```python
from build123d import *

# Parameters (mm, degrees)
SKETCH1_R                    = 241.3
SKETCH1_R_2                  = 190.5
SKETCH1_R_3                  = 12.7
BOSS_EXTRUDE1_DEPTH          = 25.4
SKETCH19_W                   = 762
SKETCH19_H                   = 609.6
BASE_FLANGE1_DEPTH           = 6
EDGE_FLANGE1_STRIP_CUT_DEPTH = 609.6
EDGE_FLANGE1_DEPTH           = 609.6
EDGE_FLANGE2_STRIP_W         = 25.4732
EDGE_FLANGE2_STRIP_H         = 6
EDGE_FLANGE2_STRIP_CUT_DEPTH = 609.6
EDGE_FLANGE2_DEPTH           = 609.6
BOSS_EXTRUDE2_DEPTH          = 12.7
BOSS_EXTRUDE2_DEPTH_BACK     = 12.7
FILLET1_R                    = 76.2
SKETCH30_R                   = 12.7
CUT_EXTRUDE1_DEPTH           = 783.174585068
FILLET3_R                    = 76.2


# Sheet-metal steps are written as plain solids
with BuildPart() as part:
    # Sketch1 → Boss-Extrude1 (new body)
    with BuildSketch(Plane.XY):
        Circle(SKETCH1_R)
        Circle(SKETCH1_R_2, mode=Mode.SUBTRACT)
        with Locations((55.879031838, 208.543385896)):
            Circle(SKETCH1_R_3, mode=Mode.SUBTRACT)
        with Locations((152.664354058, 152.664354058)):
            Circle(SKETCH1_R_3, mode=Mode.SUBTRACT)
        with Locations((208.543385896, 55.879031838)):
            Circle(SKETCH1_R_3, mode=Mode.SUBTRACT)
        with Locations((208.543385896, -55.879031838)):
            Circle(SKETCH1_R_3, mode=Mode.SUBTRACT)
        with Locations((152.664354058, -152.664354058)):
            Circle(SKETCH1_R_3, mode=Mode.SUBTRACT)
        with Locations((55.879031838, -208.543385896)):
            Circle(SKETCH1_R_3, mode=Mode.SUBTRACT)
        with Locations((-55.879031838, -208.543385896)):
            Circle(SKETCH1_R_3, mode=Mode.SUBTRACT)
        with Locations((-152.664354058, -152.664354058)):
            Circle(SKETCH1_R_3, mode=Mode.SUBTRACT)
        with Locations((-208.543385896, -55.879031838)):
            Circle(SKETCH1_R_3, mode=Mode.SUBTRACT)
        with Locations((-208.543385896, 55.879031838)):
            Circle(SKETCH1_R_3, mode=Mode.SUBTRACT)
        with Locations((-152.664354058, 152.664354058)):
            Circle(SKETCH1_R_3, mode=Mode.SUBTRACT)
        with Locations((-55.879031838, 208.543385896)):
            Circle(SKETCH1_R_3, mode=Mode.SUBTRACT)
    extrude(amount=BOSS_EXTRUDE1_DEPTH)



with BuildPart() as body_2:
    # Sketch19 → Base-Flange1 (new body)
    with BuildSketch(Plane(origin=(0, -317.5, 0), x_dir=(1, 0, 0), z_dir=(0, 1, 0))):
        with Locations((0, -12.7)):
            Rectangle(SKETCH19_W, SKETCH19_H)
    extrude(amount=-BASE_FLANGE1_DEPTH)

    # Edge-Flange1 strip (across the edge) → Edge-Flange1 strip cut (cut)
    with BuildSketch(Plane(origin=(381, -317.5, 317.5), x_dir=(-0.7071067811865438, 0.7071067811865512, 0), z_dir=(0, 0, -1))):
        Polygon((-22.039168001, 13.553886626), (-4.026895542, -4.458385832), (0.215745145, -0.215745145), (-17.796527314, 17.796527314), align=None)
    extrude(amount=EDGE_FLANGE1_STRIP_CUT_DEPTH, mode=Mode.SUBTRACT)

    # Edge-Flange1 section (across the edge) → Edge-Flange1 (add)
    with BuildSketch(Plane(origin=(381, -317.5, 317.5), x_dir=(-0.7071067811865438, 0.7071067811865512, 0), z_dir=(0, 0, -1))):
        with BuildLine():
            Line((-6, 0.30510971), (-6, 356.670718626))
            Line((-6, 356.670718626), (0, 356.670718626))
            Line((0, 356.670718626), (0, 0.30510971))
            ThreePointArc((0, 0.30510971), (0.056070336, 0.023225094), (0.215745145, -0.215745145))
            Line((0.215745145, -0.215745145), (-4.026895542, -4.458385832))
            ThreePointArc((-4.026895542, -4.458385832), (-5.487206859, -2.2728755), (-6, 0.30510971))
        make_face()
    extrude(amount=EDGE_FLANGE1_DEPTH)

    # Edge-Flange2 strip (across the edge) → Edge-Flange2 strip cut (cut)
    with BuildSketch(Plane(origin=(-381, -317.5, -292.1), x_dir=(1, 0, 0), z_dir=(0, 0, 1))):
        with Locations((-12, -3)):
            Rectangle(EDGE_FLANGE2_STRIP_W, EDGE_FLANGE2_STRIP_H)
    extrude(amount=EDGE_FLANGE2_STRIP_CUT_DEPTH, mode=Mode.SUBTRACT)

    # Edge-Flange2 section (across the edge) → Edge-Flange2 (add)
    with BuildSketch(Plane(origin=(-381, -317.5, -292.1), x_dir=(1, 0, 0), z_dir=(0, 0, 1))):
        with BuildLine():
            Line((-6, 0.7366), (-6, 248))
            Line((-6, 248), (0, 248))
            Line((0, 248), (0, 0.7366))
            ThreePointArc((0, 0.7366), (0.215745145, 0.215745145), (0.7366, 0))
            Line((0.7366, 0), (0.7366, -6))
            ThreePointArc((0.7366, -6), (-4.026895542, -4.026895542), (-6, 0.7366))
        make_face()
    extrude(amount=EDGE_FLANGE2_DEPTH)


with BuildPart() as part_1:
    add(part.part)

    add(body_2.part)  # Boss-Extrude2 merges body 2
    # Sketch2 → Boss-Extrude2 (add, two sides: drawn at the far end of the back side and taken through both)
    with BuildSketch(Plane(origin=(0, 0, 12.7), x_dir=(-1, 0, 0), z_dir=(0, 0, -1)).offset(-BOSS_EXTRUDE2_DEPTH_BACK)):
        with BuildLine():
            Line((-176.371629871, 164.677679655), (-508, -190.5))
            Line((-508, -190.5), (-381, -317.5))
            Line((-381, -317.5), (381, -317.5))
            Line((381, -317.5), (381, -190.5))
            Line((381, -190.5), (211.187529283, 116.728391899))
            ThreePointArc((211.187529283, 116.728391899), (-29.628031694, -239.474152547), (-176.371629871, 164.677679655))
        make_face()
    extrude(amount=BOSS_EXTRUDE2_DEPTH + BOSS_EXTRUDE2_DEPTH_BACK)

    # Fillet1
    # the kernel refuses this fillet: 76.2 mm, written as the material it adds along each edge
    with BuildSketch(Plane(origin=(-381, -190.5, 0), x_dir=(0, 1, 0), z_dir=(0, 0, 1))) as fillet1_piece_1:
        with BuildLine():
            CenterArc((194.419807723, -20.395387566), FILLET1_R, 164.475167034, 76.594355804)
            Line((157.558210281, -87.086186287), (156.820978332, -88.420002261))
            Line((156.820978332, -88.420002261), (-0.737231949, -1.333815974))
            Line((-0.737231949, -1.333815974), (0, 1.524))
            ThreePointArc((0, 1.524), (60.5, 1.524), (119.531603846, 0.407907751))
            Line((119.531603846, 0.407907751), (121, 0))
        make_face()
    extrude(amount=25.4)
    with BuildSketch(Plane(origin=(508, -190.5, 25.4), x_dir=(0.7071067811865509, 0.707106781186544, 0), z_dir=(0, 0, -1))) as fillet1_piece_2:
        with BuildLine():
            CenterArc((FILLET1_R * 1.03487581695, -FILLET1_R), FILLET1_R, 90, 91.963796982)
            Line((FILLET1_R * 0.0354631377737, -FILLET1_R * 1.03426801283), (FILLET1_R * 0.0154748841901, -FILLET1_R * 1.03495337309))
            Line((FILLET1_R * 0.0154748841901, -FILLET1_R * 1.03495337309), (-FILLET1_R * 0.020697516339, FILLET1_R * 0.02))
            Line((-FILLET1_R * 0.020697516339, FILLET1_R * 0.02), (FILLET1_R * 1.03487581695, FILLET1_R * 0.02))
            Line((FILLET1_R * 1.03487581695, FILLET1_R * 0.02), (FILLET1_R * 1.03487581695, 0))
        make_face()
    extrude(amount=25.4)

    # Sketch30 → Cut-Extrude1 (cut, through all)
    # profile 1 of 3: a face of its own
    with BuildSketch(Plane(origin=(0, 0, 0), x_dir=(-1, 0, 0), z_dir=(0, 0, -1))):
        with BuildLine():
            Line((-330.130702101, 0), (-241.3, 0))
            ThreePointArc((-241.3, 0), (-224.481808047, 88.507671171), (-176.371629871, 164.677679655))
            Line((-176.371629871, 164.677679655), (-330.130702101, 0))
        make_face()
    # profile 2 of 3: a face of its own
    with BuildSketch(Plane(origin=(0, 0, 0), x_dir=(-1, 0, 0), z_dir=(0, 0, -1))):
        with BuildLine():
            Line((-241.3, 0), (-190.5, 0))
            ThreePointArc((-190.5, 0), (0, 190.5), (190.5, 0))
            Line((190.5, 0), (241.3, 0))
            ThreePointArc((241.3, 0), (233.650637508, 60.274949954), (211.187529283, 116.728391899))
            ThreePointArc((211.187529283, 116.728391899), (29.628031694, 239.474152547), (-176.371629871, 164.677679655))
            ThreePointArc((-176.371629871, 164.677679655), (-224.481808047, 88.507671171), (-241.3, 0))
        make_face()
        with Locations((-208.543385896, 55.879031838)):
            Circle(SKETCH30_R, mode=Mode.SUBTRACT)
        with Locations((-152.664354058, 152.664354058)):
            Circle(SKETCH30_R, mode=Mode.SUBTRACT)
        with Locations((-55.879031838, 208.543385896)):
            Circle(SKETCH30_R, mode=Mode.SUBTRACT)
        with Locations((208.543385896, 55.879031838)):
            Circle(SKETCH30_R, mode=Mode.SUBTRACT)
        with Locations((55.879031838, 208.543385896)):
            Circle(SKETCH30_R, mode=Mode.SUBTRACT)
        with Locations((152.664354058, 152.664354058)):
            Circle(SKETCH30_R, mode=Mode.SUBTRACT)
    # profile 3 of 3: a face of its own
    with BuildSketch(Plane(origin=(0, 0, 0), x_dir=(-1, 0, 0), z_dir=(0, 0, -1))):
        with BuildLine():
            ThreePointArc((211.187529283, 116.728391899), (233.650637508, 60.274949954), (241.3, 0))
            Line((241.3, 0), (275.706099682, 0))
            Line((275.706099682, 0), (211.187529283, 116.728391899))
        make_face()
    extrude(amount=-CUT_EXTRUDE1_DEPTH, mode=Mode.SUBTRACT)

    # Fillet3
    fillet3_edges = [part_1.edges().sort_by_distance(p)[0] for p in [
        (-275.706099682, 0, 12.7),
        (330.130702101, 0, 12.7),
    ]]
    fillet(fillet3_edges, radius=FILLET3_R)


solid = part_1.part
```
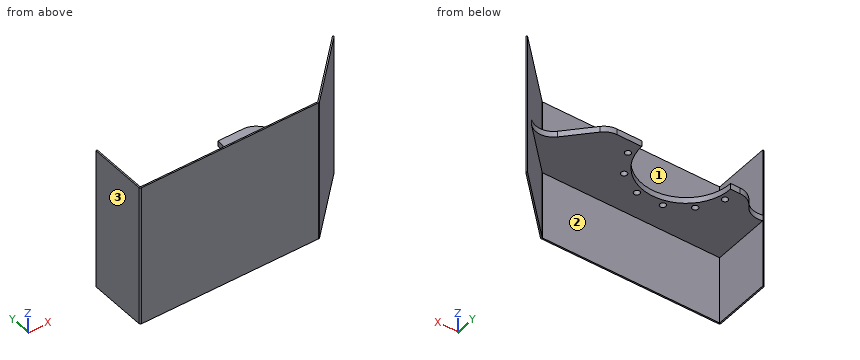
CAD build for the part. Positions are in the model's coordinates, mm. Face numbers are marked on the shaded views. A direction names the side the tool comes from. Coordinates: 2 decimals unless noted, no trailing zeros. Order: outer loops, then holes, each group sorted by start corner. A loop starts at its lowest first (then second) coordinate and runs counter-clockwise, first axis right, second up.
(1) Which spindle directions (+Z, -Z, +X, -X, +Y, -Y) get a long thin tool onto all of the face, cutting with end or side? Do the marked faces 1, 2 and 3. Say none if no direction does.
Solution:
face 1: +Z, +Y
face 2: -Z, +Y
face 3: +Z, -Z, -X, +Y, -Y
(2) Saw through at A-A, the plane x = 0. Write the cut outline in (y, z).
Solution:
outline: (-323.5, -292.1) - (-317.5, -292.1) - (-317.5, 0) - (-190.5, 0) - (-190.5, 25.4) - (-317.5, 25.4) - (-317.5, 317.5) - (-323.5, 317.5) - close
(3) Saw through at C-C, the plane x = 477.5. Write the cut outline in (y, z), and give its area (3 significant figures).
Solution:
outline: (-229.49, -292.1) - (-221, -292.1) - (-221, 0) - (-149.84, 0) - (-149.84, 25.4) - (-221, 25.4) - (-221, 317.5) - (-229.49, 317.5) - close
area: 6,980 mm2
(4) Saw through at B-B, the plane y = -241.5. Write the cut outline in (x, z).
Solution:
outline: (-387, -292.1) - (-381, -292.1) - (-381, 0) - (457, 0) - (457, -292.1) - (465.49, -292.1) - (465.49, 317.5) - (457, 317.5) - (457, 25.4) - (-381, 25.4) - (-381, 317.5) - (-387, 317.5) - close
(5) Drill centre lines: L1, parallel to Y at x = -61.5, z = -31.5; L2, parallel to Z at x = 333, y = -60; L3, parallel to X at y = -308.5, z = -257.5. Where is each one in solid material? Low to high.
Solution:
L1: y = -323.5 to -317.5
L2: z = 0 to 25.4
L3: x = -387 to -381, 390 to 398.49
(6) Pin check, flat tips, straight feed: pin 1 Ø5 at (x, y) = (257, -235) entering from +Z; pin 2 Ø8 at (x, y) = (351, -225) entering from -Z; pin 3 Ø12 at (x, z) = (429, 130) entering from +Y. Stop position of each tip, or through.
Solution:
pin 1: stops at z = 25.4
pin 2: stops at z = 0
pin 3: stops at y = -263.5
